Verification items for the finished model (mm, model axes). A direction names the side the tool comes from. Coordinates: 2 decimals unless noted, no trailing zeros. Loops run counter-clockwise (first coordinate to the right, second up) from the corner with the lowest first, then second, coordinate; pieces in that order, holes last.
Q1. Sectioned sample at C-C (z = -83). Enter the section's corners in (x, y).
Q2. Go/stop test with flat-tipped pins: P1, Ø5, axis at x = 95.5, y = 134.5, coming from the -Z side; P2, Ø8, axis at x = 122, y = 168, coming from the -Z side; P3, Ø10, axis at y = 147, z = -84.5, coming from the -X side. Record where each tip stops, or that it passes through.
Q3. Sectioned sample at B-B (x = -256). Enter the section's corners in (y, z), then the cut area to 3 significant figures.
Q4. Material ranges on probe 1 along Z at (x, y) = (140.5, 81); probe 2 along X at (y, z) = (57.5, -83.5); probe 3 along X at (y, z) = (71, -100), recorded low to high.
Q5. Access from +Z, -Z, +X, -X, +Y, -Y to the whole of each face (thin tool, end or side, straight path). Record for faces 1 (the face through (100, 123, -81)), 2 (the face through (-4, 0, -43)), 3 (the face through (-202, 123, -54)).
Q6. Sectioned sample at A-A (y = 169). Enter the section's corners in (x, z), then the cut area to 3 significant figures.
```python
from build123d import *

# Parameters (mm, degrees)
EXTRUDE_1_DEPTH = 250


with BuildPart() as part:
    # 草图1 → 凸台-拉伸1 (new body)
    with BuildSketch(Plane(origin=(0, 0, 0), x_dir=(1, 0, 0), z_dir=(0, 1, 0))):
        with BuildLine():
            Line((-297.5, 0), (297.5, 0))
            ThreePointArc((297.5, 0), (304.571067812, 2.928932188), (307.5, 10))
            Line((307.5, 10), (307.5, 44))
            ThreePointArc((307.5, 44), (304.571067812, 51.071067812), (297.5, 54))
            Line((297.5, 54), (110, 54))
            ThreePointArc((110, 54), (102.928932188, 56.928932188), (100, 64))
            Line((100, 64), (100, 98))
            ThreePointArc((100, 98), (97.071067812, 105.071067812), (90, 108))
            Line((90, 108), (-90, 108))
            ThreePointArc((-90, 108), (-97.071067812, 105.071067812), (-100, 98))
            Line((-100, 98), (-100, 64))
            ThreePointArc((-100, 64), (-102.928932188, 56.928932188), (-110, 54))
            Line((-110, 54), (-297.5, 54))
            ThreePointArc((-297.5, 54), (-304.571067812, 51.071067812), (-307.5, 44))
            Line((-307.5, 44), (-307.5, 10))
            ThreePointArc((-307.5, 10), (-304.571067812, 2.928932188), (-297.5, 0))
        make_face()
    extrude(amount=EXTRUDE_1_DEPTH)


solid = part.part
```
Geometry check:
1. outline: (-100, 0) - (100, 0) - (100, 250) - (-100, 250) - close
2. P1: stops at z = -107.54
2. P2: stops at z = -54
2. P3: stops at x = -100
3. outline: (0, -54) - (250, -54) - (250, 0) - (0, 0) - close
3. area: 13,500 mm2
4. probe 1: z = -54 to 0
4. probe 2: x = -100 to 100
4. probe 3: x = -99.8 to 99.8
5. face 1: -Z, +X, +Y, -Y
5. face 2: +Z, -Z, +X, -X, -Y
5. face 3: -Z, -X, +Y, -Y
6. outline: (-307.5, -44) arc R10 ccw to (-297.5, -54) - (-110, -54) arc R10 cw to (-100, -64) - (-100, -98) arc R10 ccw to (-90, -108) - (90, -108) arc R10 ccw to (100, -98) - (100, -64) arc R10 cw to (110, -54) - (297.5, -54) arc R10 ccw to (307.5, -44) - (307.5, -10) arc R10 ccw to (297.5, 0) - (-297.5, 0) arc R10 ccw to (-307.5, -10) - close
6. area: 43,900 mm2
